Build history of the part. All positions in model axes, mm. Round coordinates to 2 decimals unless told otherwise and drop trailing zeros. Write each loop counter-clockwise with the first axis right and the second up, starting at its lowest first coordinate (ties: lowest second). Pieces come first, ordered by that corner, then holes. Notation, with made-up numbers: M -0.5,38 L 15.5,38 A18 ccw 15.5,61 Z; hole C 42,37 d5. An arc over 180 degrees is marked long. Use a Markdown table: item, result.
from build123d import *

# Parameters (mm, degrees)
EXTRUDE1_DEPTH      = 111.76
LPATTERN1_COUNT     = 6
LPATTERN1_PITCH     = 10.16
LPATTERN1_COL_COUNT = 6
LPATTERN1_COL_PITCH = 10.16
LPATTERN2_COUNT     = 6
LPATTERN2_PITCH     = 10.16
LPATTERN2_COL_COUNT = 6
LPATTERN2_COL_PITCH = 10.16


with BuildPart() as part:
    # Sketch1 → Extrude1 (new body)
    with BuildSketch(Plane.XY):
        Polygon((0, 0), (0, 15.875), (1.5875, 15.875), (1.5875, 1.5875), (15.875, 1.5875), (15.875, 0), align=None)
    extrude(amount=EXTRUDE1_DEPTH)

    # Sketch3 → #4 Clearance Hole1 (revolve, cut)
    with BuildSketch(Plane(origin=(9.3853, 1.5875, 55.88), x_dir=(0, 0, 1), z_dir=(1, 0, 0))):
        Polygon((0, 0), (0, 16.220574487), (1.63195, 15.24), (1.63195, 0), align=None)
    f_4_clearance_hole1 = revolve(axis=Axis((9.3853, 7.9375, 55.88), (0, -1, 0)), mode=Mode.SUBTRACT)

    # LPattern1: #4 Clearance Hole1 ×6
    with Locations(*[(0, 0, i * LPATTERN1_PITCH) for i in range(1, LPATTERN1_COUNT)]):
        add(f_4_clearance_hole1, mode=Mode.SUBTRACT)

    # LPattern1 col: #4 Clearance Hole1 ×6
    with Locations(*[(0, 0, -i * LPATTERN1_COL_PITCH) for i in range(1, LPATTERN1_COL_COUNT)]):
        add(f_4_clearance_hole1, mode=Mode.SUBTRACT)

    # Sketch5 → #4 Clearance Hole2 (revolve, cut)
    with BuildSketch(Plane(origin=(1.5875, 9.3726, 55.88), x_dir=(0, 0, -1), z_dir=(0, 1, 0))):
        Polygon((0, 0), (0, 16.220574487), (1.63195, 15.24), (1.63195, 0), align=None)
    f_4_clearance_hole2 = revolve(axis=Axis((7.9375, 9.3726, 55.88), (-1, 0, 0)), mode=Mode.SUBTRACT)

    # LPattern2: #4 Clearance Hole2 ×6
    with Locations(*[(0, 0, i * LPATTERN2_PITCH) for i in range(1, LPATTERN2_COUNT)]):
        add(f_4_clearance_hole2, mode=Mode.SUBTRACT)

    # LPattern2 col: #4 Clearance Hole2 ×6
    with Locations(*[(0, 0, -i * LPATTERN2_COL_PITCH) for i in range(1, LPATTERN2_COL_COUNT)]):
        add(f_4_clearance_hole2, mode=Mode.SUBTRACT)


solid = part.part
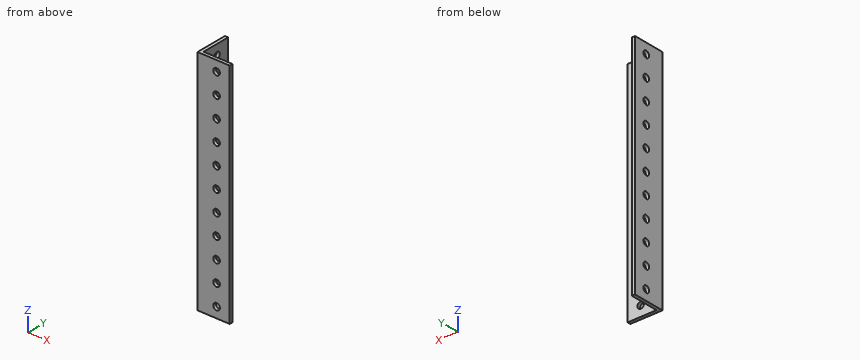
Q1. Drop flat-ended pins along their axis: P1, Ø2.5, axis at x = 9.39, z = 35.56, coming from the -Y side; P2, Ø4.5, axis at y = 10, z = 56.5, coming from the +X side; P3, Ø4, axis at x = 9.39, z = 5.08, coming from the +Y side. Give the stop position or say it passes through.
Response values:
| item | result |
|---|---|
| P1 | passes through |
| P2 | stops at x = 1.59 |
| P3 | stops at y = 1.59 |
Q2. Cut at C-C on y = 13. Give the cut face in (x, z), and give its area (3 significant figures).
Response values:
| item | result |
|---|---|
| outline | M 0,0 L 1.59,0 L 1.59,111.76 L 0,111.76 Z |
| area | 177 mm2 |
Q3. Cut at A-A on z = 35.56. Give the cut face in (x, y) (1 decimal), and give its area (3 significant figures).
Response values:
| item | result |
|---|---|
| outline | M 0,0 L 7.8,0 L 7.8,1.6 L 1.6,1.6 L 1.6,7.7 L 0,7.7 Z; M 0,11 L 1.6,11 L 1.6,15.9 L 0,15.9 Z; M 11,0 L 15.9,0 L 15.9,1.6 L 11,1.6 Z |
| area | 37.5 mm2 |
Q4. Drill centre lines: L1, parallel to Y at x = 1, z = 106.68 (3 decimals); L2, parallel to X at y = 0.5, z = 86.36 (3 decimals); L3, parallel to Y at x = 4.25, z = 56. Where is each one in solid material? Low to high.
Response values:
| item | result |
|---|---|
| L1 | y = 0 to 7.741, 11.005 to 15.875 |
| L2 | x = 0 to 7.753, 11.017 to 15.875 |
| L3 | y = 0 to 1.59 |
Q5. Cut at B-B on z = 103. Give the cut face in (x, y) (1 decimal).
Response values:
| item | result |
|---|---|
| outline | M 0,0 L 15.9,0 L 15.9,1.6 L 1.6,1.6 L 1.6,15.9 L 0,15.9 Z |
